```python
from build123d import *

# Parameters (mm, degrees)
BOSS_EXTRUDE1_DEPTH        = 12.7
F_10_32_TAPPED_HOLE1_D     = 4.0386
F_10_32_TAPPED_HOLE1_DEPTH = 25.4
F_10_32_TAPPED_HOLE1_TIP   = 1.213317848
F_10_32_TAPPED_HOLE2_D     = 4.0386
F_10_32_TAPPED_HOLE2_DEPTH = 25.4
F_10_32_TAPPED_HOLE2_TIP   = 1.213317848


with BuildPart() as part:
    # Sketch1 → Boss-Extrude1 (new body)
    with BuildSketch(Plane(origin=(0, 0, 0), x_dir=(1, 0, 0), z_dir=(0, 1, 0))):
        Polygon((-25.4, -25.4), (25.4, 25.4), (25.4, -25.4), align=None)
    extrude(amount=BOSS_EXTRUDE1_DEPTH)

    # #10-32 Tapped Hole1
    with Locations(Plane(origin=(25.4, 0, 0), x_dir=(0, 0, -1), z_dir=(1, 0, 0))):
        with Locations((6.35, 6.35)):
            Hole(F_10_32_TAPPED_HOLE1_D / 2, depth=F_10_32_TAPPED_HOLE1_DEPTH)
            with Locations((0, 0, -(F_10_32_TAPPED_HOLE1_DEPTH + F_10_32_TAPPED_HOLE1_TIP / 2))):  # 118° drill point
                Cone(0, F_10_32_TAPPED_HOLE1_D / 2, F_10_32_TAPPED_HOLE1_TIP, mode=Mode.SUBTRACT)

    # #10-32 Tapped Hole2
    with Locations(Plane.XY.offset(25.4)):
        with Locations((-6.35, 6.35)):
            Hole(F_10_32_TAPPED_HOLE2_D / 2, depth=F_10_32_TAPPED_HOLE2_DEPTH)
            with Locations((0, 0, -(F_10_32_TAPPED_HOLE2_DEPTH + F_10_32_TAPPED_HOLE2_TIP / 2))):  # 118° drill point
                Cone(0, F_10_32_TAPPED_HOLE2_D / 2, F_10_32_TAPPED_HOLE2_TIP, mode=Mode.SUBTRACT)


solid = part.part
```
Model file for the job. Use its own axes, mm. Give positions to 0.01 mm unless a question says otherwise; leave off trailing zeros. Order: outer loops, then holes, each group sorted by start corner. A loop starts at its lowest first (then second) coordinate and runs counter-clockwise, first axis right, second up.
1) Saw through at C-C, the plane z = -6.35. Write the cut outline in (x, y).
2) Pin check, flat tips, straight feed: pin 1 (5.5 mm diameter, centred on y = 6.35, z = -6.35, fed in from -X); pin 2 (5.5 mm diameter, centred on x = -6.35, y = 6.35, fed in from -Z); pin 3 (3 mm diameter, centred on x = -4.5, y = 6, fed in from -Z). Stop position of each tip, or through.
3) Mould opens along Z. For faces 1 (the cylindrical face through (14.718, 6.957, -4.424)), 2 (the flat face through (0, 6, 0)), 3 (the flat face through (12, 12.7, 11)) say: +Z half, -Z half, draft (parallel to the pull), parting line (faces both ways), or undercut.
4) Saw through at D-D, the plane z = 11. Write the cut outline in (x, y), then the cut area to 3 significant figures.
5) Wall check: probe 1 along Y at (x, z) = (-6.35, 15); probe 2 along X at (y, z) = (4.5, 22); probe 3 along X at (y, z) = (6.35, 16.25). Give the ranges that are in metal, low to high.
6) Saw through at A-A, the plane x = -6.35. Write the cut outline in (y, z).
7) Saw through at B-B, the plane y = 6.35. Write the cut outline in (x, z).
Computed:
1. outline: (6.35, 0) - (25.4, 0) - (25.4, 4.33) - (6.35, 4.33) - close; (6.35, 8.37) - (25.4, 8.37) - (25.4, 12.7) - (6.35, 12.7) - close
2. pin 1: stops at x = 3.6
2. pin 2: stops at z = 3.6
2. pin 3: stops at z = 3
3. face 1: undercut
3. face 2: -Z half
3. face 3: draft
4. outline: (-11, 0) - (25.4, 0) - (25.4, 12.7) - (-11, 12.7) - close; hole circle Ø4.04 at (-6.35, 6.35)
4. area: 449 mm2
5. probe 1: y = 0 to 4.33, 8.37 to 12.7
5. probe 2: x = -22 to -7.16, -5.54 to 25.4
5. probe 3: x = -16.25 to -8.37, -4.33 to 25.4
6. outline: (0, 6.35) - (4.33, 6.35) - (4.33, 25.4) - (0, 25.4) - close; (8.37, 6.35) - (12.7, 6.35) - (12.7, 25.4) - (8.37, 25.4) - close
7. outline: (-25.4, 25.4) - (-8.37, 8.37) - (-8.37, 25.4) - close; (-4.33, 4.33) - (4.33, -4.33) - (25.4, -4.33) - (25.4, 25.4) - (-4.33, 25.4) - close; (8.37, -8.37) - (25.4, -25.4) - (25.4, -8.37) - close
